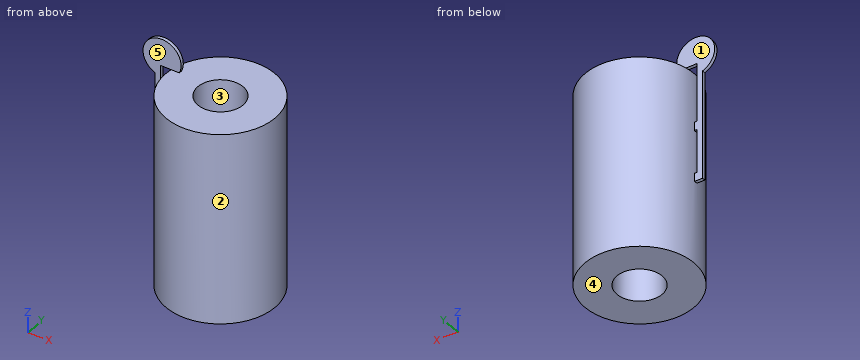
from build123d import *

# Parameters (mm, degrees)
F0_W     = 50
F0_H     = 175
F2_R     = 20.721056
F3_DEPTH = 235
F5_DEPTH = 3


with BuildPart() as f1:
    # F0 (on Front) → F1 (revolve)
    with BuildSketch(Plane.XZ):
        with Locations((1.541793, 32.918449)):
            Rectangle(F0_W, F0_H)
    revolve(axis=Axis((26.541793, 0, 32.918449), (0, 0, -1)))

    # F2 (on face) → F3 (cut)
    with BuildSketch(Plane.XY.offset(120.418449)):
        with Locations((26.541793, 0)):
            Circle(F2_R)
    extrude(amount=-F3_DEPTH, mode=Mode.SUBTRACT)

    # F4 (on Front) → F5 (join)
    with BuildSketch(Plane.XZ):
        with BuildLine():
            Line((-30.847115, 20.86447), (-23.65957, 20.86447))
            Line((-23.65957, 20.86447), (-23.131855, 28.351171))
            Line((-23.131855, 28.351171), (-25.822921, 28.351171))
            Line((-25.822921, 28.351171), (-25.822921, 67.948289))
            Line((-25.822921, 67.948289), (-23.131855, 67.948289))
            Line((-23.131855, 67.948289), (-23.131855, 75.637057))
            Line((-23.131855, 75.637057), (-25.822921, 75.637057))
            Line((-25.822921, 75.637057), (-25.822921, 128.891826))
            Line((-25.822921, 128.891826), (-8.927411, 128.891826))
            ThreePointArc((-8.927411, 128.891826), (-31.173128, 152.219995), (-30.847115, 119.986951))
            Line((-30.847115, 119.986951), (-30.847115, 20.86447))
        make_face()
    extrude(amount=F5_DEPTH)


solid = f1.part
Verification items for the finished model (mm, model axes). Face numbers are marked on the shaded views. A direction names the side the tool comes from. Coordinates: 2 decimals unless noted, no trailing zeros. Order: outer loops, then holes, each group sorted by start corner. A loop starts at its lowest first (then second) coordinate and runs counter-clockwise, first axis right, second up.
Item 1: Material ranges on L1, parallel to Z at x = 36, y = 42; L2, parallel to Y at x = 44, z = -40; L3, parallel to X at y = -6, z = 29.5, recorded low to high.
Filled in:
L1: z = -54.58 to 120.42
L2: y = -46.85 to -11.16, 11.16 to 46.85
L3: x = -23.1 to 6.71, 46.38 to 76.18
Item 2: Section check A-A, the plane z = 48.5. Enter the section's corners in (x, y), then the cut area to 3 significant figures.
Filled in:
outline: (-30.85, -3) - (-25.82, -3) - (-25.82, 0) - (-30.85, 0) - close; circle Ø100 at (26.54, 0); hole circle Ø41.44 at (26.54, 0)
area: 6,520 mm2
Item 3: Depth check by flat-ended pin: pin 1 (12 mm diameter, centred on x = 36.5, z = 7, fed in from +Y); pin 2 (10 mm diameter, centred on x = 39, y = -37, fed in from +Z); pin 3 (1.5 mm diameter, centred on y = -1, z = 102, fed in from +X). Enter the tip coordinate at first touch or a pass-through.
Filled in:
pin 1: stops at y = 49.84
pin 2: stops at z = 120.42
pin 3: stops at x = 76.54
Item 4: Section check B-B, the plane x = -11.5. Enter the section's corners in (y, z).
Filled in:
outline: (-32.45, -54.58) - (32.45, -54.58) - (32.45, 120.42) - (-32.45, 120.42) - close; (-3, 128.89) - (0, 128.89) - (0, 147.45) - (-3, 147.45) - close
Item 5: Access from +Z, -Z, +X, -X, +Y, -Y to the whole of each face (thin tool, end or side, straight path). Record for the marked faces 4 and 5.
Filled in:
face 4: -Z, +X, -X, +Y, -Y
face 5: +Z, -X, -Y
Item 6: Section check C-C, the plane z = -2. Enter the section's corners in (x, y), then the cut area to 3 significant figures.
Filled in:
outline: circle Ø100 at (26.54, 0); hole circle Ø41.44 at (26.54, 0)
area: 6,510 mm2
Item 7: Release check for a two-part mould opening along Y. For the marked faces 1, 2 and 3 record: +Y half, -Y half, draft (parallel to the pull), parting line (faces both ways), or undercut.
Filled in:
face 1: +Y half
face 2: parting line
face 3: undercut
Item 8: Section check D-D, the plane x = 38. Enter the section's corners in (y, z), then the cut area to 3 significant figures.
Filled in:
outline: (-48.67, -54.58) - (-17.26, -54.58) - (-17.26, 120.42) - (-48.67, 120.42) - close; (17.26, -54.58) - (48.67, -54.58) - (48.67, 120.42) - (17.26, 120.42) - close
area: 11,000 mm2
